from build123d import *

# Parameters (mm, degrees)
SKETCH_1_W             = 160
SKETCH_1_H             = 66
EXTRUDE_1_DEPTH        = 18.5
SKETCH_2_R             = 25
CUT_EXTRUDE_1_DEPTH    = 20
HOLE_WIZARD_M6_1_D     = 5
PATTERN_LINEAR_1_COUNT = 4
PATTERN_LINEAR_1_PITCH = 15
CUT_EXTRUDE_4_DEPTH    = 40
HOLE_WIZARD_M4_1_D     = 3.3
HOLE_WIZARD_M4_1_DEPTH = 10.1
HOLE_WIZARD_M4_1_TIP   = 0.991420021


with BuildPart() as part:
    # 草图1 → 凸台-拉伸1 (new body)
    with BuildSketch(Plane.XY):
        with Locations((80, 33)):
            Rectangle(SKETCH_1_W, SKETCH_1_H)
    extrude(amount=EXTRUDE_1_DEPTH)

    # 草图2 → 切除-拉伸1 (cut)
    with BuildSketch(Plane.XY.offset(18.5)):
        with Locations((-0.1, 33)):
            Circle(SKETCH_2_R)
    extrude(amount=-CUT_EXTRUDE_1_DEPTH, mode=Mode.SUBTRACT)

    # M6 螺纹孔1 (through all)
    with Locations(Plane(origin=(0, 0, 0), x_dir=(-1, 0, 0), z_dir=(0, 0, -1))):
        with Locations((-147, 53), (-147, 13)):
            hole_wizard_m6_1 = Hole(HOLE_WIZARD_M6_1_D / 2)

    # 阵列(线性)1: M6 螺纹孔1 ×4
    with Locations(*[(-i * PATTERN_LINEAR_1_PITCH, 0, 0) for i in range(1, PATTERN_LINEAR_1_COUNT)]):
        add(hole_wizard_m6_1, mode=Mode.SUBTRACT)

    # 草图7 → 切除-拉伸4 (cut)
    with BuildSketch(Plane(origin=(0, 0, 0), x_dir=(-1, 0, 0), z_dir=(0, 0, -1))):
        with BuildLine():
            Line((-30, 49.75), (-58, 49.75))
            ThreePointArc((-58, 49.75), (-61.25, 53), (-58, 56.25))
            Line((-58, 56.25), (-30, 56.25))
            ThreePointArc((-30, 56.25), (-26.75, 53), (-30, 49.75))
        make_face()
        with BuildLine():
            Line((-30, 16.25), (-58, 16.25))
            ThreePointArc((-58, 16.25), (-61.25, 13), (-58, 9.75))
            Line((-58, 9.75), (-30, 9.75))
            ThreePointArc((-30, 9.75), (-26.75, 13), (-30, 16.25))
        make_face()
    extrude(amount=-CUT_EXTRUDE_4_DEPTH, mode=Mode.SUBTRACT)

    # M4 螺纹孔1
    with Locations(Plane.ZY):
        with Locations((4.75, 5), (13.75, 5), (4.75, 61), (13.75, 61)):
            Hole(HOLE_WIZARD_M4_1_D / 2, depth=HOLE_WIZARD_M4_1_DEPTH)
            with Locations((0, 0, -(HOLE_WIZARD_M4_1_DEPTH + HOLE_WIZARD_M4_1_TIP / 2))):  # 118° drill point
                Cone(0, HOLE_WIZARD_M4_1_D / 2, HOLE_WIZARD_M4_1_TIP, mode=Mode.SUBTRACT)


solid = part.part
Can you work these out from the model? Positions are in its coordinate system, mm. A direction names the side the tool comes from. Give positions to 0.01 mm unless a question says otherwise; leave off trailing zeros. Order: outer loops, then holes, each group sorted by start corner. A loop starts at its lowest first (then second) coordinate and runs counter-clockwise, first axis right, second up. Notation, with made-up numbers: M 51,30 L 74,30 A22 ccw 74,49 Z; hole C 11,62 d6. An arc over 180 degrees is marked long. Use one line per item in the form item = value.
Item 1: If we section it at B-B, the plane y = 53: Write out the boundary of the cut face in (x, z).
Values follow:
outline = M 14.9,0 L 26.75,0 L 26.75,18.5 L 14.9,18.5 Z; M 61.25,0 L 99.5,0 L 99.5,18.5 L 61.25,18.5 Z; M 104.5,0 L 114.5,0 L 114.5,18.5 L 104.5,18.5 Z; M 119.5,0 L 129.5,0 L 129.5,18.5 L 119.5,18.5 Z; M 134.5,0 L 144.5,0 L 144.5,18.5 L 134.5,18.5 Z; M 149.5,0 L 160,0 L 160,18.5 L 149.5,18.5 Z
Item 2: Will these pins go through, and if not, where does the flat tip stop? pin 1 Ø6 at (x, y) = (102, 53) entering from +Z; pin 2 Ø3 at (x, y) = (117, 53) entering from -Z; pin 3 Ø1.5 at (y, z) = (44, 7) entering from -X; pin 4 Ø4 at (y, z) = (36, 11) entering from -X.
Values follow:
pin_1 = 18.5
pin_2 = through
pin_3 = 21.97
pin_4 = 24.39
Item 3: If I drill on line 1 along Y through (x, z) = (102, 6); line 2 along Y through (x, z) = (32, 6.75); line 3 along Z through (x, y) = (5.75, 61), over which ranges is the centre line in solid material (lowest first)? Write a range as [from, to].
Values follow:
line_1 = [0, 10.5], [15.5, 50.5], [55.5, 66]
line_2 = [0, 9.75], [16.25, 49.75], [56.25, 66]
line_3 = [0, 3.1], [6.4, 12.1], [15.4, 18.5]
Item 4: For faces 4 (the cylindrical face through (5.12, 4, 6.06)), 5 (the cylindrical face through (26.75, 12.93, 9.12)), 6 (the flat face through (79, 33, 18.5)), which set-ups out of +Z, -Z, +X, -X, +Y, -Y let a thin tool reach every point of the face, with its end or its side?
Values follow:
face_4 = -X
face_5 = +Z, -Z
face_6 = +Z, +X, -X, +Y, -Y
Item 5: Thinking about a two-plate mould opening in Y: for faces 1 (the flat face through (44, 56.25, 9)), 2 (the flat face through (0, 62, 9)), 3 (the flat face through (79, 0, 9)), which applies, pulls with the +Y half, pulls with the -Y half, needs draft (parallel to the pull), parting line crosses it, or undercut?
Values follow:
face_1 = undercut
face_2 = needs draft
face_3 = pulls with the -Y half
Item 6: If we section it at D-D, the plane y = 26: Write out the boundary of the cut face in (x, z).
Values follow:
outline = M 23.9,0 L 160,0 L 160,18.5 L 23.9,18.5 Z
Item 7: If we section it at C-C, the plane x = 55: Write out the boundary of the cut face in (y, z).
Values follow:
outline = M 0,0 L 9.75,0 L 9.75,18.5 L 0,18.5 Z; M 16.25,0 L 49.75,0 L 49.75,18.5 L 16.25,18.5 Z; M 56.25,0 L 66,0 L 66,18.5 L 56.25,18.5 Z
Item 8: If we section it at A-A, the plane x = 117: Write out the boundary of the cut face in (y, z).
Values follow:
outline = M 0,0 L 10.5,0 L 10.5,18.5 L 0,18.5 Z; M 15.5,0 L 50.5,0 L 50.5,18.5 L 15.5,18.5 Z; M 55.5,0 L 66,0 L 66,18.5 L 55.5,18.5 Z
